from build123d import *

# Parameters (mm, degrees)
SKETCH1_W            = 26.3
SKETCH1_H            = 14.05
BOSS_EXTRUDE6_DEPTH  = 1
SKETCH5_W            = 24.3
SKETCH5_H            = 1
BOSS_EXTRUDE8_DEPTH  = 10.05
SKETCH6_W            = 26.3
SKETCH6_H            = 27.07
SKETCH6_W_2          = 24.3
SKETCH6_H_2          = 12.05
BOSS_EXTRUDE9_DEPTH  = 2.5
SKETCH7_R            = 1.8
CUT_EXTRUDE1_DEPTH   = 2.5
SKETCH8_W            = 4.4
SKETCH8_H            = 5
CUT_EXTRUDE2_DEPTH   = 2.5
CUT_EXTRUDE3_DEPTH   = 2.5
SKETCH10_W           = 12
SKETCH10_H           = 8
CUT_EXTRUDE5_DEPTH   = 2.5
SKETCH11_W           = 2
SKETCH11_H           = 7
CUT_EXTRUDE7_DEPTH   = 2.5
SKETCH12_W           = 2
SKETCH12_H           = 3
BOSS_EXTRUDE11_DEPTH = 1
SKETCH13_W           = 2
SKETCH13_H           = 8
BOSS_EXTRUDE14_DEPTH = 1
SKETCH14_W           = 2
SKETCH14_H           = 4
BOSS_EXTRUDE15_DEPTH = 1.4
SKETCH15_W           = 12.05
SKETCH15_H           = 10.05
CUT_EXTRUDE8_DEPTH   = 1.4
SKETCH16_W           = 2
SKETCH16_H           = 3
CUT_EXTRUDE9_DEPTH   = 1.4


with BuildPart() as part:
    # Sketch1 → Boss-Extrude6 (new body)
    with BuildSketch(Plane(origin=(0, 0, 0), x_dir=(1, 0, 0), z_dir=(0, 1, 0))):
        with Locations((13.15, 7.025)):
            Rectangle(SKETCH1_W, SKETCH1_H)
    extrude(amount=BOSS_EXTRUDE6_DEPTH)

    # Sketch5 → Boss-Extrude8 (add)
    with BuildSketch(Plane(origin=(0, 1, 0), x_dir=(1, 0, 0), z_dir=(0, 1, 0))):
        with Locations((13.15, 13.55)):
            Rectangle(SKETCH5_W, SKETCH5_H)
        Polygon((26.3, 14.05), (25.3, 14.05), (25.3, 13.05), (25.3, 1), (25.3, 0), (26.3, 0), align=None)
        with Locations((13.15, 0.5)):
            Rectangle(SKETCH5_W, SKETCH5_H)
        Polygon((1, 14.05), (0, 14.05), (0, 0), (1, 0), (1, 1), (1, 13.05), align=None)
    extrude(amount=BOSS_EXTRUDE8_DEPTH)

    # Sketch6 → Boss-Extrude9 (add)
    with BuildSketch(Plane(origin=(0, 11.05, 0), x_dir=(1, 0, 0), z_dir=(0, 1, 0))):
        with Locations((13.15, 7.025)):
            Rectangle(SKETCH6_W, SKETCH6_H)
        with Locations((13.15, 7.025)):
            Rectangle(SKETCH6_W_2, SKETCH6_H_2, mode=Mode.SUBTRACT)
    extrude(amount=-BOSS_EXTRUDE9_DEPTH)

    # Sketch7 → Cut-Extrude1 (cut)
    with BuildSketch(Plane(origin=(0, 11.05, 0), x_dir=(1, 0, 0), z_dir=(0, 1, 0))):
        with Locations(Location((6, -3.26, 0), (0, 0, 270))):
            Circle(SKETCH7_R)
        with Locations(Location((20.3, -3.26, 0), (0, 0, 270))):
            Circle(SKETCH7_R)
        with Locations(Location((6, 17.31, 0), (0, 0, 270))):
            Circle(SKETCH7_R)
        with Locations(Location((20.3, 17.31, 0), (0, 0, 270))):
            Circle(SKETCH7_R)
    extrude(amount=-CUT_EXTRUDE1_DEPTH, mode=Mode.SUBTRACT)

    # Sketch8 → Cut-Extrude2 (cut)
    with BuildSketch(Plane(origin=(26.3, 0, 0), x_dir=(0, 0, -1), z_dir=(1, 0, 0))):
        with Locations((7.025, 8.55)):
            Rectangle(SKETCH8_W, SKETCH8_H)
    extrude(amount=-CUT_EXTRUDE2_DEPTH, mode=Mode.SUBTRACT)

    # Sketch9 → Cut-Extrude3 (cut)
    with BuildSketch(Plane(origin=(26.3, 0, 0), x_dir=(0, 0, -1), z_dir=(1, 0, 0))):
        with BuildLine():
            Line((9.225, 6.05), (4.825, 6.05))
            ThreePointArc((4.825, 6.05), (7.025, 3.85), (9.225, 6.05))
        make_face()
    extrude(amount=-CUT_EXTRUDE3_DEPTH, mode=Mode.SUBTRACT)

    # Sketch10 → Cut-Extrude5 (cut)
    with BuildSketch(Plane.XZ):
        with Locations((8.5, -7.025)):
            Rectangle(SKETCH10_W, SKETCH10_H)
    extrude(amount=-CUT_EXTRUDE5_DEPTH, mode=Mode.SUBTRACT)

    # Sketch11 → Cut-Extrude7 (cut)
    with BuildSketch(Plane.ZY):
        with Locations((-3.5, 7.55)):
            Rectangle(SKETCH11_W, SKETCH11_H)
        with Locations((-10.55, 7.55)):
            Rectangle(SKETCH11_W, SKETCH11_H)
    extrude(amount=-CUT_EXTRUDE7_DEPTH, mode=Mode.SUBTRACT)

    # Sketch12 → Boss-Extrude11 (add)
    with BuildSketch(Plane.ZY):
        with Locations((-3.5, 9.55)):
            Rectangle(SKETCH12_W, SKETCH12_H)
        with Locations((-10.55, 9.55)):
            Rectangle(SKETCH12_W, SKETCH12_H)
    extrude(amount=-BOSS_EXTRUDE11_DEPTH)

    # Sketch13 → Boss-Extrude14 (add)
    with BuildSketch(Plane.XZ):
        with Locations((3.5, -7.025)):
            Rectangle(SKETCH13_W, SKETCH13_H)
    extrude(amount=-BOSS_EXTRUDE14_DEPTH)

    # Sketch14 → Boss-Extrude15 (add)
    with BuildSketch(Plane.ZY):
        Polygon((-20.56, 8.55), (-14.05, 8.55), (-14.05, 0), (0, 0), (0, 8.55), (6.51, 8.55), (6.51, 11.05), (-20.56, 11.05), align=None)
        with Locations((-10.55, 6.05)):
            Rectangle(SKETCH14_W, SKETCH14_H, mode=Mode.SUBTRACT)
        with Locations((-3.5, 6.05)):
            Rectangle(SKETCH14_W, SKETCH14_H, mode=Mode.SUBTRACT)
    extrude(amount=BOSS_EXTRUDE15_DEPTH)

    # Sketch15 → Cut-Extrude8 (cut)
    with BuildSketch(Plane(origin=(1, 0, 0), x_dir=(0, 0, -1), z_dir=(1, 0, 0))):
        with Locations((7.025, 6.025)):
            Rectangle(SKETCH15_W, SKETCH15_H)
    extrude(amount=-CUT_EXTRUDE8_DEPTH, mode=Mode.SUBTRACT)

    # Sketch16 → Cut-Extrude9 (cut)
    with BuildSketch(Plane.ZY.offset(1.4)):
        with Locations((-10.55, 9.55)):
            Rectangle(SKETCH16_W, SKETCH16_H)
        with Locations((-3.5, 9.55)):
            Rectangle(SKETCH16_W, SKETCH16_H)
    extrude(amount=-CUT_EXTRUDE9_DEPTH, mode=Mode.SUBTRACT)


solid = part.part
Geometry check sheet. Reference: the model listing, model coordinates, mm. A direction names the side the tool comes from. Coordinates: 2 decimals unless noted, no trailing zeros. Order: outer loops, then holes, each group sorted by start corner. A loop starts at its lowest first (then second) coordinate and runs counter-clockwise, first axis right, second up. Notation, with made-up numbers: (-32, 57) - (-10, 57) arc R10 cw to (-10, 76) - close; hole circle Ø8 at (8, 54.5). An arc over 180 degrees is marked (long way). Answer in a Markdown table with one row per item. Add a question column.
1) Cross-section at A-A, the plane x = 20.3. Record the cut outline in (y, z), then the cut area to 3 significant figures.
2) Gauge pin test, flat ends, axial feed: P1, Ø0.5, axis at x = -1, y = 6.5, coming from the +Z side; P2, Ø3, axis at x = 12, y = 3, coming from the -Z side; P3, Ø3.5, axis at x = 16.5, z = -6, coming from the +Y side; P4, Ø5, axis at y = 3, z = 3.5, coming from the +X side. Record the tip position at first contact, or that the pin passes through.
3) Set-up check for faces 1 (the flat face through (-1, 8, -4.5)), 2 (the flat face through (26, 9, -9.225)), 3 (the flat face through (9.4, 0.5, -3.025)), 4 (the flat face through (13, 4, 0)): record each of +Z, -Z, +X, -X, +Y, -Y from which the full face is reachable in a straight line by a thin tool's end or side.
4) Release check for a two-part mould opening along X. For faces 5 (the cylindrical face through (25.81, 3.85, -6.98)), 6 (the flat face through (26.3, 3, -7)), 7 (the flat face through (15, 1, -7)), 8 (the cylindrical face through (18.543, 9.818, 2.87)) record: +X half, -X half, draft (parallel to the pull), parting line (faces both ways), or undercut.
5) Cross-section at C-C, the plane y = 8. Record the cut outline in (x, z) (3 decimals).
6) Cross-section at B-B, the plane x = 11.25. Record the cut outline in (y, z) (3 decimals).
7) Cross-section at D-D, the plane z = -10. Record the cut outline in (x, y), then the cut area to 3 significant figures.
8) Material ranges on line 1 along X through (y, z) = (10.2, 3.26); line 2 along Z through (x, y) = (6.25, 6.5); line 3 along X through (y, z) = (3, -10), recorded low to high. Write a range as [from, to].
Check result:
| question | item | result |
|---|---|---|
| 1 | outline | (0, -14.05) - (8.55, -14.05) - (8.55, -15.51) - (11.05, -15.51) - (11.05, -13.05) - (1, -13.05) - (1, -1) - (11.05, -1) - (11.05, 1.46) - (8.55, 1.46) - (8.55, 0) - (0, 0) - close; (8.55, -20.56) - (11.05, -20.56) - (11.05, -19.11) - (8.55, -19.11) - close; (8.55, 5.06) - (11.05, 5.06) - (11.05, 6.51) - (8.55, 6.51) - close |
| 1 | area | 48.7 mm² |
| 2 | P1 | stops at z = 0 |
| 2 | P2 | stops at z = -14.05 |
| 2 | P3 | stops at y = 1 |
| 2 | P4 | passes through |
| 3 | face 1 | -X, +Y |
| 3 | face 2 | +X, +Y |
| 3 | face 3 | +Y, -Y |
| 3 | face 4 | +Z, +X, -X, -Y |
| 4 | face 5 | draft |
| 4 | face 6 | +X half |
| 4 | face 7 | undercut |
| 4 | face 8 | undercut |
| 5 | outline | (-1.4, -14.05) - (26.3, -14.05) - (26.3, -9.225) - (25.3, -9.225) - (25.3, -13.05) - (-0.4, -13.05) - (-0.4, -11.55) - (-1.4, -11.55) - close; (-1.4, -9.55) - (-0.4, -9.55) - (-0.4, -4.5) - (-1.4, -4.5) - close; (-1.4, -2.5) - (-0.4, -2.5) - (-0.4, -1) - (25.3, -1) - (25.3, -4.825) - (26.3, -4.825) - (26.3, 0) - (-1.4, 0) - close |
| 6 | outline | (0, -14.05) - (8.55, -14.05) - (8.55, -20.56) - (11.05, -20.56) - (11.05, -13.05) - (1, -13.05) - (1, -11.025) - (0, -11.025) - close; (0, -3.025) - (1, -3.025) - (1, -1) - (11.05, -1) - (11.05, 6.51) - (8.55, 6.51) - (8.55, 0) - (0, 0) - close |
| 7 | outline | (-1.4, 0) - (4.5, 0) - (4.5, 1) - (-0.4, 1) - (-0.4, 4.05) - (-1.4, 4.05) - close; (14.5, 0) - (26.3, 0) - (26.3, 11.05) - (25.3, 11.05) - (25.3, 1) - (14.5, 1) - close |
| 7 | area | 30.8 mm² |
| 8 | line 1 | x = [-1.4, 4.2], [7.8, 18.5], [22.1, 26.3] |
| 8 | line 2 | z = [-14.05, -13.05], [-1, 0] |
| 8 | line 3 | x = [-1.4, -0.4], [25.3, 26.3] |
